For this review, take the finished solid that the model builds, in its own axes (mm). Face numbers are marked on the shaded views. A direction names the side the tool comes from. Coordinates: 2 decimals unless noted, no trailing zeros. Loops run counter-clockwise (first coordinate to the right, second up) from the corner with the lowest first, then second, coordinate; pieces in that order, holes last. Notation, with made-up numbers: (31, 22.25) - (42, 22.25) arc R15 cw to (42, 32.25) - close; hole circle Ø8 at (37.5, 66.5). An arc over 180 degrees is marked (long way). One line per item, written item: value. Start each with the question number.
1. The part is to be moulded in two halves that separate along X. For the marked faces 3, 4 and 5, say which applies: released by +X, released by -X, zero draft, split by the parting line, or undercut.
2. Take a section at B-B, the plane y = 37. State the section outline as (x, z) points.
3. To check wall thickness, follow line 1 (Y direction, x = 14, z = 7.25); line 2 (X direction, y = 37, z = 6.5); line 3 (Z direction, x = 11.5, y = 21). State the ranges of each line that lie inside material, in increasing order. Write a range as from..to.
4. Take a section at C-C, the plane x = 14. State the section outline as (y, z) points.
5. Take a section at A-A, the plane z = 7.25. State the section outline as (x, y) points, and give its area (3 significant figures).
6. For the marked faces 1 and 2, list the 3-axis set-ups (+Z, -Z, +X, -X, +Y, -Y) from which the entire face can be reached by the end or side of a thin tool; tool diameter is ignored.
7. Insertion check: pin 1 (1.4 mm diameter, centred on x = 12.5, y = 38.5, fed in from +Z). The pin has a flat end and moves straight along its axis. Give the tip position at first contact, or say it passes through.
```python
from build123d import *

# Parameters (mm, degrees)
BOX001_W     = 12
BOX001_H     = 4.7
BOX001_DEPTH = 11
BOX002_W     = 12
BOX002_H     = 4.7
BOX002_DEPTH = 11
BOX_W        = 12
BOX_H        = 4.7
BOX_DEPTH    = 11
BOX003_W     = 21
BOX003_H     = 45
BOX003_DEPTH = 10


with BuildPart() as box001:
    # Box001 → Box001 (new body)
    with BuildSketch(Plane(origin=(0, 15, 0), x_dir=(1, 0, 0), z_dir=(0, 0, 1))):
        with Locations((6, 2.35)):
            Rectangle(BOX001_W, BOX001_H)
    extrude(amount=BOX001_DEPTH)


with BuildPart() as box002:
    # Box002 → Box002 (new body)
    with BuildSketch(Plane(origin=(0, 30, 0), x_dir=(1, 0, 0), z_dir=(0, 0, 1))):
        with Locations((6, 2.35)):
            Rectangle(BOX002_W, BOX002_H)
    extrude(amount=BOX002_DEPTH)


with BuildPart() as ranuras:
    # Box → Box (new body)
    with BuildSketch(Plane.XY):
        with Locations((6, 2.35)):
            Rectangle(BOX_W, BOX_H)
    extrude(amount=BOX_DEPTH)

    # Fusion: union Box001, Box002
    add(box001.part)
    add(box002.part)


with BuildPart() as ranuras_1:
    # Fusion placement: moved
    add(ranuras.part.moved(Location((5, 5, 3))))


with BuildPart() as porta_pendrives:
    # Box003 → Box003 (new body)
    with BuildSketch(Plane.XY):
        with Locations((10.5, 22.5)):
            Rectangle(BOX003_W, BOX003_H)
    extrude(amount=BOX003_DEPTH)

    # Cut: cut Ranuras
    add(ranuras_1.part, mode=Mode.SUBTRACT)


solid = porta_pendrives.part
```
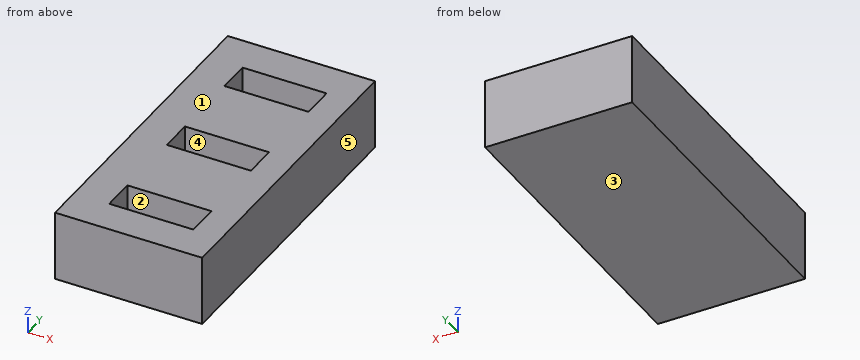
Solutions:
1. face 3: zero draft
1. face 4: undercut
1. face 5: released by +X
2. outline: (0, 0) - (21, 0) - (21, 10) - (17, 10) - (17, 3) - (5, 3) - (5, 10) - (0, 10) - close
3. line 1: 0..5, 9.7..20, 24.7..35, 39.7..45
3. line 2: 0..5, 17..21
3. line 3: 0..3
4. outline: (0, 0) - (45, 0) - (45, 10) - (39.7, 10) - (39.7, 3) - (35, 3) - (35, 10) - (24.7, 10) - (24.7, 3) - (20, 3) - (20, 10) - (9.7, 10) - (9.7, 3) - (5, 3) - (5, 10) - (0, 10) - close
5. outline: (0, 0) - (21, 0) - (21, 45) - (0, 45) - close; hole (5, 5) - (17, 5) - (17, 9.7) - (5, 9.7) - close; hole (5, 20) - (17, 20) - (17, 24.7) - (5, 24.7) - close; hole (5, 35) - (17, 35) - (17, 39.7) - (5, 39.7) - close
5. area: 776 mm2
6. face 1: +Z, +X, -X, +Y, -Y
6. face 2: +Z
7. pin 1: z = 3
